from build123d import *

# Parameters (mm, degrees)
BOSS_EXTRUDE1_DEPTH = 9
SKETCH2_R           = 1.0922
CUT_EXTRUDE1_DEPTH  = 10


with BuildPart() as part:
    # Sketch1 → Boss-Extrude1 (new body)
    with BuildSketch(Plane.XY):
        Polygon((3.129243729, 7.05753004), (2.129243729, 7.05753004), (2.129243729, -22.94246996), (3.129243729, -22.94246996), (3.129243729, -4.94246996), align=None)
    extrude(amount=BOSS_EXTRUDE1_DEPTH)

    # Sketch2 → Cut-Extrude1 (cut)
    with BuildSketch(Plane(origin=(3.129243729, 0, 0), x_dir=(0, 0, -1), z_dir=(1, 0, 0))):
        with Locations(Location((-4.5, 0.89753004, 0), (0, 0, 90))):
            Circle(SKETCH2_R)
        with Locations(Location((-4.5, -16.78246996, 0), (0, 0, 90))):
            Circle(SKETCH2_R)
    extrude(amount=-CUT_EXTRUDE1_DEPTH, mode=Mode.SUBTRACT)


solid = part.part
Design review of the part built by this model. Coordinates are the model's own, in mm. Coordinates: 2 decimals unless noted, no trailing zeros. Order: outer loops, then holes, each group sorted by start corner. A loop starts at its lowest first (then second) coordinate and runs counter-clockwise, first axis right, second up. Notation, with made-up numbers: M -22.5,-4 L -18.5,-4 A23 ccw -18.5,4 Z; hole C 4,71.25 d2. An arc over 180 degrees is marked long. Use a Markdown table: item, result.
(1) Add section C-C (x = 2.95). Give the boundary of the cut face in (y, z).
Worked answers:
| item | result |
|---|---|
| outline | M -22.94,0 L 7.06,0 L 7.06,9 L -22.94,9 Z; hole C -16.78,4.5 d2.18; hole C 0.9,4.5 d2.18 |
(2) Wall thickness on probe 1 along Y at (x, z) = (2.55, 5.25); probe 2 along Z at (x, y) = (2.65, 1.75); probe 3 along Z at (x, y) = (2.45, 0.25): over which ranges is each line inside the solid? List them lowest first.
Worked answers:
| item | result |
|---|---|
| probe 1 | y = -22.94 to -17.58, -15.99 to 0.1, 1.69 to 7.06 |
| probe 2 | z = 0 to 3.82, 5.18 to 9 |
| probe 3 | z = 0 to 3.62, 5.38 to 9 |
(3) Add section B-B (y = 1.5). Give the boundary of the cut face in (x, z).
Worked answers:
| item | result |
|---|---|
| outline | M 2.13,0 L 3.13,0 L 3.13,3.59 L 2.13,3.59 Z; M 2.13,5.41 L 3.13,5.41 L 3.13,9 L 2.13,9 Z |
(4) Draft analysis for pull direction Y (two halves, no side actions). For faces 1 (the flat face through (2.6, -7.7, 0)), 2 (the flat face through (2.6, -22.942, 4.4)), 3 (the cylindrical face through (2.636, -17.649, 3.835)), state which applies: released by +Y, released by -Y, zero draft, split by the parting line, or undercut.
Worked answers:
| item | result |
|---|---|
| face 1 | zero draft |
| face 2 | released by -Y |
| face 3 | undercut |
(5) Add section A-A (z = 4.5). Give the boundary of the cut face in (x, y), then the cut area to 3 significant figures.
Worked answers:
| item | result |
|---|---|
| outline | M 2.13,-22.94 L 3.13,-22.94 L 3.13,-17.87 L 2.13,-17.87 Z; M 2.13,-15.69 L 3.13,-15.69 L 3.13,-0.19 L 2.13,-0.19 Z; M 2.13,1.99 L 3.13,1.99 L 3.13,7.06 L 2.13,7.06 Z |
| area | 25.6 mm2 |
(6) For P1, Ø1.7, axis at y = -16.78, z = 4.5, coming from the +X side, flat-tipped, find the tip position at first contact; note if it passes through.
Worked answers:
| item | result |
|---|---|
| P1 | passes through |
